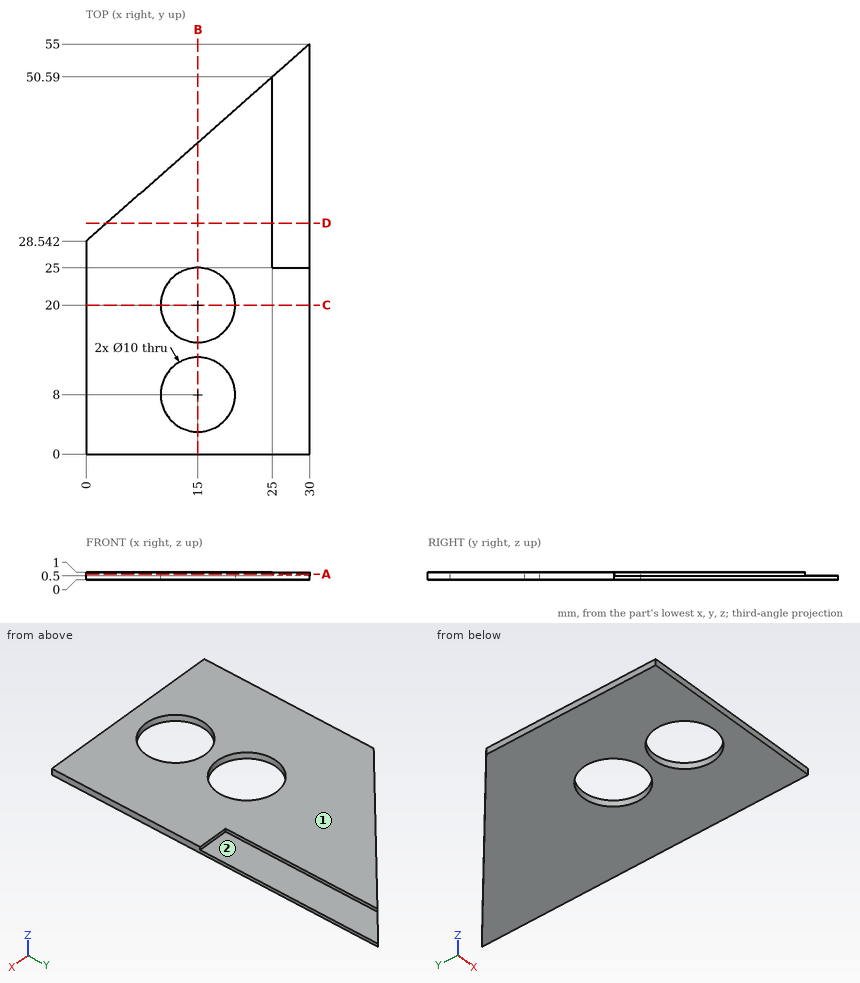
The figure shows three views and two pictorial views of one solid part (mm, origin at its lowest corner). Answer the questions. A direction names the side the tool comes from. Coordinates: 2 decimals unless noted, no trailing zeros. Write each loop counter-clockwise with the first axis right and the second up, starting at its lowest first coordinate (ties: lowest second). Pieces come first, ordered by that corner, then holes. Notation, with made-up numbers: (68.25, 34) -> (122.25, 34) arc R8 cw to (122.25, 47) -> close; hole circle Ø1 at (-34.75, 78.5). An arc over 180 degrees is marked (long way). Return JSON: item names as keys, results as strings.
1. Find the intervals of material crossed by line 1 along Y through (x, z) = (15, 0.7); line 2 along Y through (x, z) = (18, 0.8) (1 decimal); line 3 along X through (y, z) = (8.5, 0.9) (1 decimal), in increasing order. Write a range as from..to.
Found:
{"line 1": "0..3, 13..15, 25..41.77", "line 2": "0..4, 12..16, 24..44.4", "line 3": "0..10, 20..30"}
2. A cutting plane is placed at C-C (y = 20). Determine the outline of the cut face in (x, z).
Found:
{"outline": "(0, 0) -> (10, 0) -> (10, 1) -> (0, 1) -> close; (20, 0) -> (30, 0) -> (30, 1) -> (20, 1) -> close"}
3. A cutting plane is placed at A-A (z = 0.75). Determine the outline of the cut face in (x, y), and give its area (3 significant figures).
Found:
{"outline": "(0, 0) -> (30, 0) -> (30, 25) -> (25, 25) -> (25, 50.59) -> (0, 28.54) -> close; hole circle Ø10 at (15, 8); hole circle Ø10 at (15, 20)", "area": "957 mm2"}
4. This flat-tipped pin is pushed along its axis until it touches: P1, Ø0.6, axis at x = 28.5, z = 0.5, coming from the +Y side. Where does it stop, or does it pass through?
Found:
{"P1": "y = 53.94"}
5. A tool of negligible diameter and unlimited length cuts with its end or side. For the marked faces 1 and 2, from which of +Z, -Z, +X, -X, +Y, -Y can it reach the whole face along a straight path? Write none if from no direction.
Found:
{"face 1": "+Z, +X, -X, +Y, -Y", "face 2": "+Z, +X, +Y"}
6. A cutting plane is placed at D-D (y = 31). Determine the outline of the cut face in (x, z).
Found:
{"outline": "(2.79, 0) -> (30, 0) -> (30, 0.5) -> (25, 0.5) -> (25, 1) -> (2.79, 1) -> close"}
7. A cutting plane is placed at B-B (x = 15). Determine the outline of the cut face in (y, z).
Found:
{"outline": "(0, 0) -> (3, 0) -> (3, 1) -> (0, 1) -> close; (13, 0) -> (15, 0) -> (15, 1) -> (13, 1) -> close; (25, 0) -> (41.77, 0) -> (41.77, 1) -> (25, 1) -> close"}
